Check sheet for the modelled part. Datum: model origin and axes. Units: mm. Face numbers are marked on the shaded views. Give positions to 0.01 mm unless a question says otherwise; leave off trailing zeros. Order: outer loops, then holes, each group sorted by start corner. A loop starts at its lowest first (then second) coordinate and runs counter-clockwise, first axis right, second up.
Item 1: Sectioned sample at A-A on x = 0. Record the boundary of the cut face in (y, z), and give its area (3 significant figures).
Item 2: Release check for a two-part mould opening along Y. For the marked faces 1, 2, 3 and 4 record: released by +Y, released by -Y, zero draft, split by the parting line, or undercut.
Item 3: Sectioned sample at B-B on y = 0. Record the boundary of the cut face in (x, z), and give its area (3 significant figures).
Item 4: Sectioned sample at C-C on z = -0.15. Record the boundary of the cut face in (x, y).
Item 5: Material ranges on line 1 along Y through (x, z) = (0, -0.6); line 2 along X through (y, z) = (1.3, -2.1); line 3 along Z through (x, y) = (0, -0.1), recorded low to high.
Item 6: Gauge pin test, flat ends, axial feed: P1, Ø1, axis at x = 1, y = 1, coming from the +Z side; P2, Ø1.5, axis at y = 0, z = -2.5, coming from the -X side; P3, Ø1, axis at x = 4, y = 0.5, coming from the -Z side. Record the tip position at first contact, or that the pin passes through.
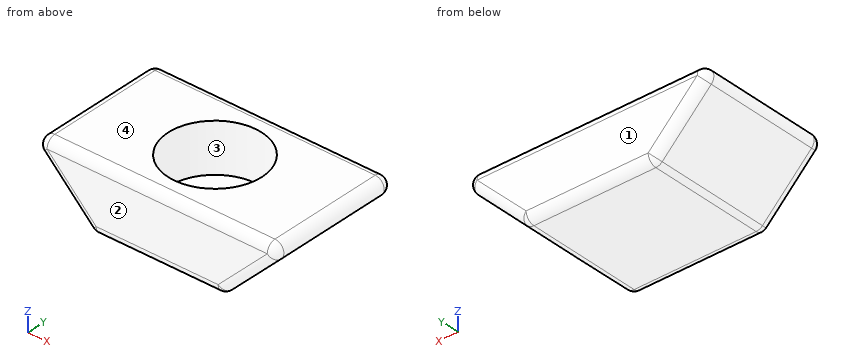
from build123d import *

# Parameters (mm, degrees)
EXTRUDE_1_DEPTH     = 3
SKETCH_3_R          = 2.1
CUT_EXTRUDE_1_DEPTH = 2.2
FILLET_1_R          = 0.4


with BuildPart() as part:
    # 草图2 → 凸台-拉伸1 (new body, symmetric)
    with BuildSketch(Plane(origin=(0, 0, 0), x_dir=(1, 0, 0), z_dir=(0, 1, 0))):
        Polygon((-5.9, 0), (5.9, 0), (2.9, 3), (-2.9, 3), align=None)
    extrude(amount=EXTRUDE_1_DEPTH, both=True)

    # 草图3 → 切除-拉伸1 (cut)
    with BuildSketch(Plane.XY):
        Circle(SKETCH_3_R)
    extrude(amount=-CUT_EXTRUDE_1_DEPTH, mode=Mode.SUBTRACT)

    # 圆角1
    fillet_1_edges = [part.edges().sort_by_distance(p)[0] for p in [
        (4.4, 3, -1.5),
        (0, 3, -3),
        (-4.4, 3, -1.5),
        (0, -3, -3),
        (4.4, -3, -1.5),
        (0, -3, 0),
        (-4.4, -3, -1.5),
        (-2.9, 0, -3),
        (2.9, 0, -3),
        (5.9, 0, 0),
        (-5.9, 0, 0),
        (0, 3, 0),
    ]]
    fillet(fillet_1_edges, radius=FILLET_1_R)


solid = part.part
Report:
1. outline: (-3, -2.6) arc R0.4 ccw to (-2.6, -3) - (2.6, -3) arc R0.4 ccw to (3, -2.6) - (3, -0.4) arc R0.4 ccw to (2.6, 0) - (2.1, 0) - (2.1, -2.2) - (-2.1, -2.2) - (-2.1, 0) - (-2.6, 0) arc R0.4 ccw to (-3, -0.4) - close
1. area: 8.62 mm2
2. face 1: released by +Y
2. face 2: released by -Y
2. face 3: undercut
2. face 4: zero draft
3. outline: (-5.22, -0.68) - (-3.02, -2.88) arc R0.4 ccw to (-2.73, -3) - (2.73, -3) arc R0.4 ccw to (3.02, -2.88) - (5.22, -0.68) arc R0.4 ccw to (4.93, 0) - (2.1, 0) - (2.1, -2.2) - (-2.1, -2.2) - (-2.1, 0) - (-4.93, 0) arc R0.4 ccw to start
3. area: 16.8 mm2
4. outline: (-5.25, -2.6) arc R0.31 ccw to (-4.93, -2.91) - (4.93, -2.91) arc R0.31 ccw to (5.25, -2.6) - (5.25, 2.6) arc R0.31 ccw to (4.93, 2.91) - (-4.93, 2.91) arc R0.31 ccw to (-5.25, 2.6) - close; hole circle Ø4.2 at (0, 0)
5. line 1: y = -3 to -2.1, 2.1 to 3
5. line 2: x = -3.8 to -1.65, 1.65 to 3.8
5. line 3: z = -3 to -2.2
6. P1: stops at z = -2.2
6. P2: stops at x = -4.15
6. P3: stops at z = -2.4
